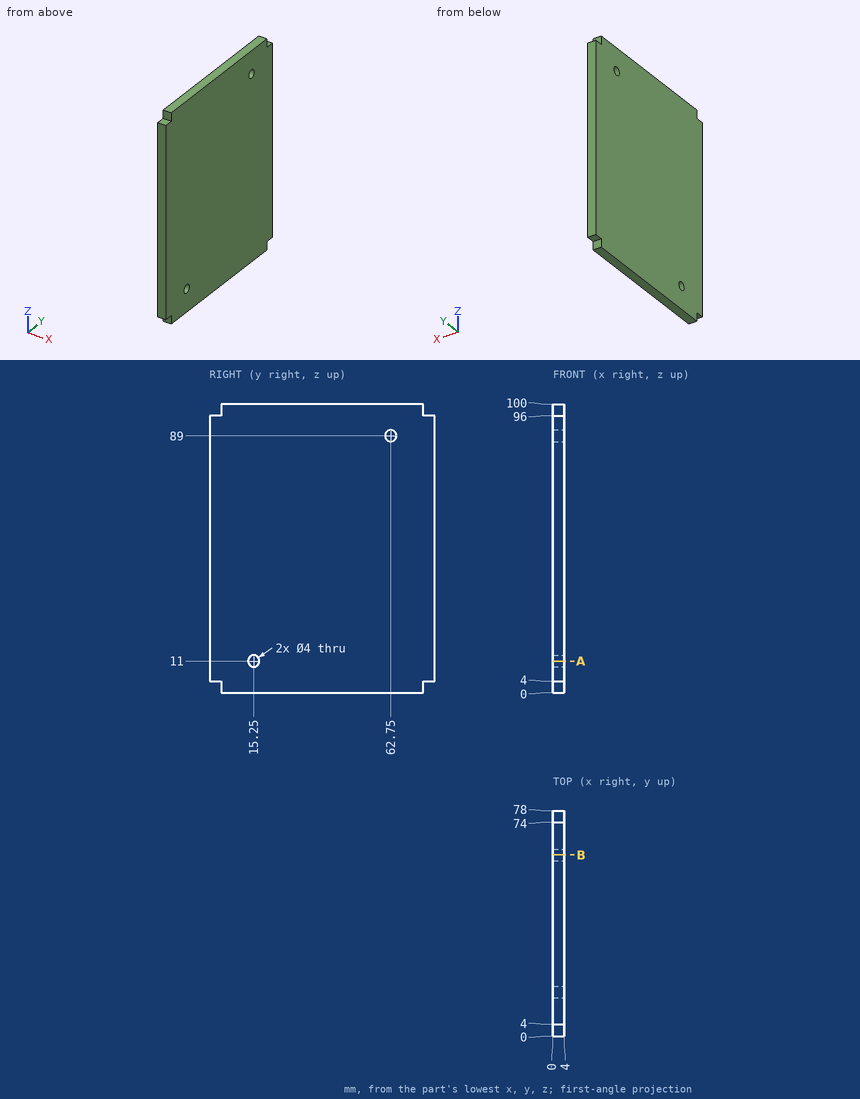
Geometry: see drawing. Coordinates: mm, zero at the bounding-box minimum. Round coordinates to 2 decimals unless told otherwise and drop trailing zeros. Loops run counter-clockwise (first coordinate to the right, second up) from the corner with the lowest first, then second, coordinate; pieces in that order, holes last. Notation, with made-up numbers: (60.25, 82.5) - (65.25, 82.5) arc R28 cw to (65.25, 106.5) - close; hole circle Ø9 at (2.5, 86). An arc over 180 degrees is marked (long way). One line per item, written item: value. Start each with the question number.
(1) Section B-B, the plane y = 62.75. Return loops of the section in (x, z).
(2) Contact query for flat-ended pins moving along their axis: P1, Ø1.2, axis at x = 1, z = 3, coming from the -Y side; P2, Ø1.2, axis at x = 2.5, y = 2, coming from the -Z side. Output: stop coordinate, or through.
(3) Ray query, line 1 (Y direction, x = 1.9, z = 11); line 2 (Y direction, x = 2.1, z = 89); line 3 (Z direction, x = 1, y = 15.25). Return the intervals inside material, ascending. Write a range as [from, to].
(4) Section A-A, the plane z = 11. Return loops of the section in (x, y).
Results below:
1. outline: (0, 0) - (4, 0) - (4, 87) - (0, 87) - close; (0, 91) - (4, 91) - (4, 100) - (0, 100) - close
2. P1: y = 4
2. P2: z = 4
3. line 1: [0, 13.25], [17.25, 78]
3. line 2: [0, 60.75], [64.75, 78]
3. line 3: [0, 9], [13, 100]
4. outline: (0, 0) - (4, 0) - (4, 13.25) - (0, 13.25) - close; (0, 17.25) - (4, 17.25) - (4, 78) - (0, 78) - close
